from build123d import *

# Parameters (mm, degrees)
F0_R     = 19.685
F2_DEPTH = 16.51
F1_R     = 10.16
F3_DEPTH = 12.7
F4_R     = 1.905
F5_DEPTH = 25.4
F6_R     = 18.415
F6_R_2   = 10.31875
F7_DEPTH = 15.24
F8_R     = 3.175
F8_R_2   = 1.905
F9_DEPTH = 8.89


with BuildPart() as f2:
    # F0 (on Front) → F2 (new body)
    with BuildSketch(Plane.XZ):
        Circle(F0_R)
    extrude(amount=-F2_DEPTH)

    # F1 (on face) → F3 (cut)
    with BuildSketch(Plane.XZ):
        Circle(F1_R)
    extrude(amount=-F3_DEPTH, mode=Mode.SUBTRACT)

    # F4 (on face) → F5 (cut)
    with BuildSketch(Plane.XZ.offset(-12.7)):
        with Locations((0, 5.715)):
            Circle(F4_R)
        with Locations((4.041115, 4.041115)):
            Circle(F4_R)
        with Locations((5.715, 0)):
            Circle(F4_R)
        with Locations((4.041115, -4.041115)):
            Circle(F4_R)
        with Locations((0, -5.715)):
            Circle(F4_R)
        with Locations((-4.041115, -4.041115)):
            Circle(F4_R)
        with Locations((-4.041115, 4.041115)):
            Circle(F4_R)
        with Locations((-5.715, 0)):
            Circle(F4_R)
    extrude(amount=-F5_DEPTH, mode=Mode.SUBTRACT)

    # F6 (on face) → F7 (cut)
    with BuildSketch(Plane(origin=(0, 16.51, 0), x_dir=(-1, 0, 0), z_dir=(0, 1, 0))):
        Circle(F6_R)
        Circle(F6_R_2, mode=Mode.SUBTRACT)
    extrude(amount=-F7_DEPTH, mode=Mode.SUBTRACT)

    # F8 (on face) → F9 (join)
    with BuildSketch(Plane(origin=(0, 16.51, 0), x_dir=(-1, 0, 0), z_dir=(0, 1, 0))):
        Circle(F8_R)
        Circle(F8_R_2, mode=Mode.SUBTRACT)
    extrude(amount=F9_DEPTH)


solid = f2.part
Work out the finished part from the listing and answer in its coordinate system (mm). A direction names the side the tool comes from. Round coordinates to 2 decimals unless told otherwise and drop trailing zeros. Order: outer loops, then holes, each group sorted by start corner. A loop starts at its lowest first (then second) coordinate and runs counter-clockwise, first axis right, second up. Notation, with made-up numbers: M 62,-39.75 L 69,-39.75 A32 ccw 69,-11.75 Z; hole C -17,30.5 d5. An arc over 180 degrees is marked long. Put each result on its own line as item: value. Start each with the question number.
Q1. A tool of negligible diameter and unlimited length cuts with its end or side. For faces 4 (the cylindrical face through (0.41, 20.89, -1.86)), 5 (the cylindrical face through (-1.323, 6.261, 10.074)), 6 (the cylindrical face through (-0.248, 14.578, -3.826)), from which of +Z, -Z, +X, -X, +Y, -Y can it reach the whole face along a straight path? Write none if from no direction.
Q2. Section D-D, the plane x = 5 is taken. Write down the section's boundary in (y, z), and give its area (3 significant figures).
Q3. Straight lines are drawn through the part: L1, parallel to Z at x = 0, y = 13.6 (3 decimals); L2, parallel to X at y = 12.25, z = 4.5; L3, parallel to X at y = 7.5, z = 8.5. For each, find the intervals that lie inside material, in ascending order. Write a range as [from, to].
Q4. For a pull along X with two mould halves and no side action, classify faces 1 (the cylindrical face through (14.61, 9, -11.21)), 2 (the flat face through (11.6, 16.51, -14.5)), 3 (the cylindrical face through (0.69, 20.89, -3.1)) as pulls with the +X half, pulls with the -X half, needs draft (parallel to the pull), parting line crosses it, or undercut.
Q5. Flat-ended cylindrical pins translate along their axes: pin 1 (2.5 mm diameter, centred on x = 0, z = -5.715, fed in from -Y); pin 2 (3 mm diameter, centred on x = -12.5, z = -10, fed in from +Y); pin 3 (3 mm diameter, centred on y = 7.5, z = -9, fed in from -X); pin 4 (1.1 mm diameter, centred on x = 0.5, z = -0.5, fed in from +Y). Find the tip coordinate at first contact, or state that the pin passes through.
Q6. Section C-C, the plane y = 7.25 is taken. Write down the section's boundary in (x, z) (1 decimal).
Q7. Section A-A, the plane x = 0 is taken. Give the number of separate pieces and of enclosed holes in the cut face, and give its area (3 significant figures).
Findings below:
1. face 4: +Y
1. face 5: -Y
1. face 6: +Y, -Y
2. outline: M 0,-19.04 L 16.51,-19.04 L 16.51,-17.72 L 1.27,-17.72 L 1.27,-9.03 L 16.51,-9.03 L 16.51,-5.69 L 12.7,-5.69 L 12.7,-8.84 L 0,-8.84 Z; M 0,8.84 L 12.7,8.84 L 12.7,5.69 L 16.51,5.69 L 16.51,9.03 L 1.27,9.03 L 1.27,17.72 L 16.51,17.72 L 16.51,19.04 L 0,19.04 Z; M 12.7,-2.4 L 16.51,-2.4 L 16.51,-1.77 L 12.7,-1.77 Z; M 12.7,1.77 L 16.51,1.77 L 16.51,2.4 L 12.7,2.4 Z
2. area: 100 mm^2
3. L1: z = [-19.685, -18.415], [-10.319, -7.62], [-3.81, 3.81], [7.62, 10.319], [18.415, 19.685]
3. L2: x = [-19.16, -17.86], [-9.29, -9.11], [9.11, 9.29], [17.86, 19.16]
3. L3: x = [-17.76, -16.34], [-5.85, -5.57], [5.57, 5.85], [16.34, 17.76]
4. face 1: undercut
4. face 2: needs draft
4. face 3: parting line crosses it
5. pin 1: passes through
5. pin 2: stops at y = 1.27
5. pin 3: stops at x = -18.2
5. pin 4: stops at y = 16.51
6. outline: C 0,0 d39.4; C 0,0 d20.6; hole C 0,0 d36.8; hole C 0,0 d20.3
7. separate pieces: 3
7. enclosed holes: 0
7. area: 139 mm^2
